Drawing for the job (mm, zero at the part's lowest x, y, z). Give positions to 0.01 mm unless a question says otherwise; leave off trailing zeros. Order: outer loops, then holes, each group sorted by start corner. A loop starts at its lowest first (then second) coordinate and runs counter-clockwise, first axis right, second up. Notation, with made-up numbers: (66, 74) - (87, 74) arc R7 cw to (87, 86) - close; hole circle Ø4 at (0, 69.25). An arc over 180 degrees is marked (long way). One line per item, written item: value.
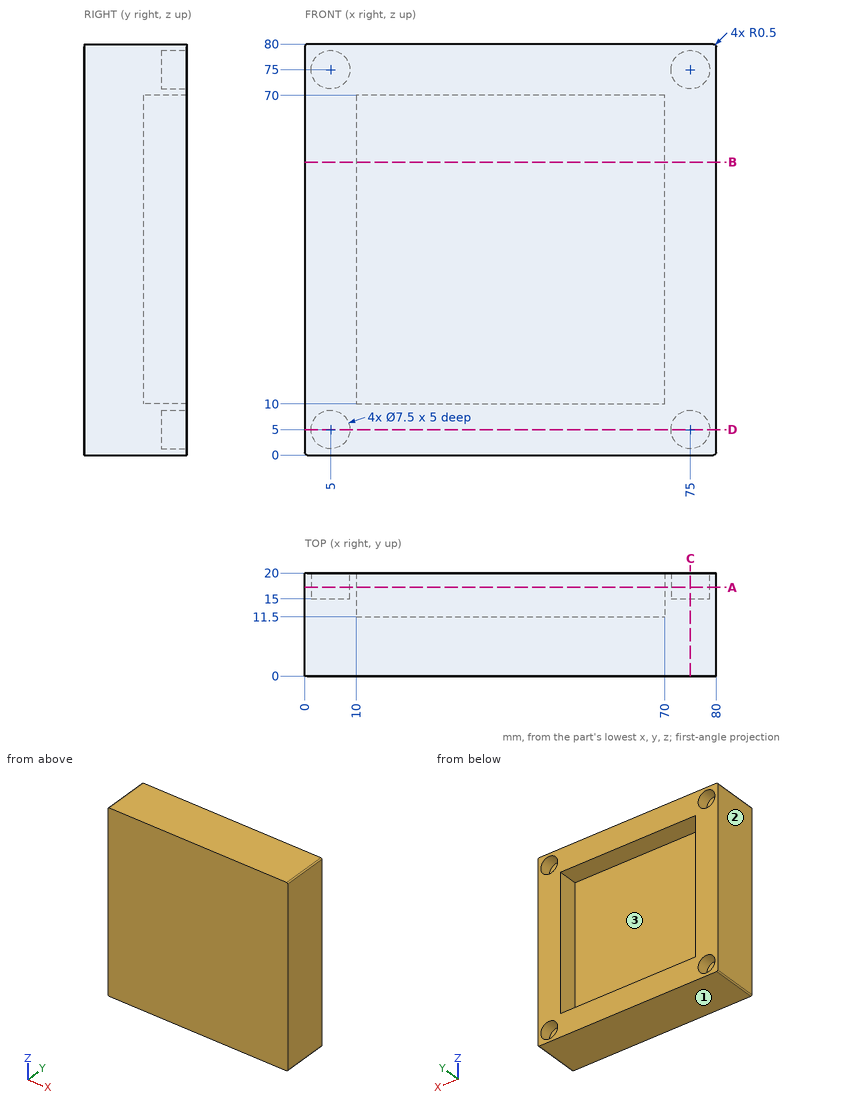
(1) Pin check, flat tips, straight feed: P1, Ø6, axis at x = 5, z = 75, coming from the +Y side; P2, Ø5, axis at x = 18, z = 15, coming from the +Y side. Stop position of each tip, or through.
Completed:
P1: y = 15
P2: y = 11.5
(2) Pull direction Z, two halves, no side cores. Call the marked faces 1, 2 and 3: +Z half, -Z half, draft (parallel to the pull), parting line (faces both ways), or undercut.
Completed:
face 1: -Z half
face 2: draft
face 3: undercut
(3) Slice it at D-D, the plane z = 5. Give the cut face in (x, y), and give its area (4 significant figures).
Completed:
outline: (0, 0) - (80, 0) - (80, 20) - (78.75, 20) - (78.75, 15) - (71.25, 15) - (71.25, 20) - (8.75, 20) - (8.75, 15) - (1.25, 15) - (1.25, 20) - (0, 20) - close
area: 1,525 mm²
(4) Drill centre lines: line 1 (Z direction, x = 5, y = 18); line 2 (X direction, y = 19, z = 42). Where is each one in solid material? Low to high.
Completed:
line 1: 0 to 1.25, 8.75 to 71.25, 78.75 to 80
line 2: 0 to 10, 70 to 80
(5) Slice it at C-C, the plane x = 75. Give the cut face in (y, z).
Completed:
outline: (0, 0) - (20, 0) - (20, 1.25) - (15, 1.25) - (15, 8.75) - (20, 8.75) - (20, 71.25) - (15, 71.25) - (15, 78.75) - (20, 78.75) - (20, 80) - (0, 80) - close
(6) Slice it at B-B, the plane z = 57. Give the cut face in (x, y), and give its area (3 significant figures).
Completed:
outline: (0, 0) - (80, 0) - (80, 20) - (70, 20) - (70, 11.5) - (10, 11.5) - (10, 20) - (0, 20) - close
area: 1,090 mm²
(7) Slice it at A-A, the plane y = 17.25. Give the cut face in (x, z), and give its area (3 significant figures).
Completed:
outline: (0, 0.5) arc R0.5 ccw to (0.5, 0) - (79.5, 0) arc R0.5 ccw to (80, 0.5) - (80, 79.5) arc R0.5 ccw to (79.5, 80) - (0.5, 80) arc R0.5 ccw to (0, 79.5) - close; hole circle Ø7.5 at (5, 5); hole circle Ø7.5 at (5, 75); hole (10, 10) - (70, 10) - (70, 70) - (10, 70) - close; hole circle Ø7.5 at (75, 5); hole circle Ø7.5 at (75, 75)
area: 2,620 mm²
